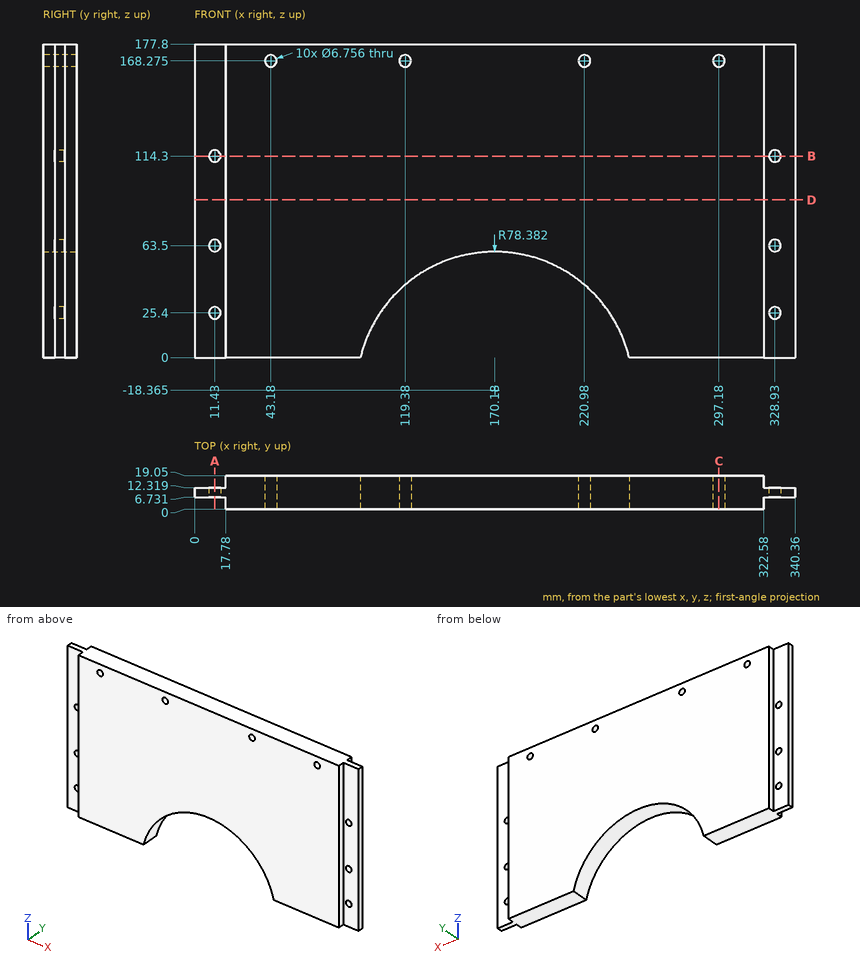
Here's the drawing with two shaded views (mm, measured from the low corner). I have some questions. Give positions to 0.01 mm unless a question says otherwise; leave off trailing zeros. Loops run counter-clockwise (first coordinate to the right, second up) from the corner with the lowest first, then second, coordinate; pieces in that order, holes last. Notation, with made-up numbers: (24.5, -10.5) -> (31.5, -10.5) arc R18 cw to (31.5, 4.5) -> close; hole circle Ø2 at (9, 16.25). An arc over 180 degrees is marked (long way). Answer as a JSON object with one key per item and string values. Group by question number.
Item 1: Imagine slicing it at A-A on x = 11.43. Write out the boundary of the cut face in (y, z).
Item 2: Imagine slicing it at C-C on x = 297.18. Write out the boundary of the cut face in (y, z).
Item 3: I need wall thicknesses on L1, parallel to Z at x = 328.93, y = 10.95; L2, parallel to Z at x = 297.18, y = 12; L3, parallel to X at y = 10, z = 167.5. Which ranges of each line are inside material? Lowest first, please.
Item 4: Imagine slicing it at B-B on z = 114.3. Write out the boundary of the cut face in (x, y).
Item 5: Will these pins go through, and if not, where does the flat tip stop? pin 1 (19.5 mm diameter, centred on x = 4.5, z = 94.5, fed in from +Y); pin 2 (3.5 mm diameter, centred on y = 15, z = 117.5, fed in from +X); pin 3 (2 mm diameter, centred on y = 3, z = 68, fed in from -X).
Item 6: Imagine slicing it at D-D on z = 89.5. Write out the boundary of the cut face in (x, y).
Answer list:
{
 "1": {"outline": "(6.73, 0) -> (12.32, 0) -> (12.32, 22.02) -> (6.73, 22.02) -> close; (6.73, 28.78) -> (12.32, 28.78) -> (12.32, 60.12) -> (6.73, 60.12) -> close; (6.73, 66.88) -> (12.32, 66.88) -> (12.32, 110.92) -> (6.73, 110.92) -> close; (6.73, 117.68) -> (12.32, 117.68) -> (12.32, 177.8) -> (6.73, 177.8) -> close"},
 "2": {"outline": "(0, 0) -> (19.05, 0) -> (19.05, 164.9) -> (0, 164.9) -> close; (0, 171.65) -> (19.05, 171.65) -> (19.05, 177.8) -> (0, 177.8) -> close"},
 "3": {"L1": "z = 0 to 22.02, 28.78 to 60.12, 66.88 to 110.92, 117.68 to 177.8", "L2": "z = 0 to 164.9, 171.65 to 177.8", "L3": "x = 0 to 39.89, 46.47 to 116.09, 122.67 to 217.69, 224.27 to 293.89, 300.47 to 340.36"},
 "4": {"outline": "(0, 6.73) -> (8.05, 6.73) -> (8.05, 12.32) -> (0, 12.32) -> close; (14.81, 6.73) -> (17.78, 6.73) -> (17.78, 0) -> (322.58, 0) -> (322.58, 6.73) -> (325.55, 6.73) -> (325.55, 12.32) -> (322.58, 12.32) -> (322.58, 19.05) -> (17.78, 19.05) -> (17.78, 12.32) -> (14.81, 12.32) -> close; (332.31, 6.73) -> (340.36, 6.73) -> (340.36, 12.32) -> (332.31, 12.32) -> close"},
 "5": {"pin 1": "stops at y = 12.32", "pin 2": "stops at x = 322.58", "pin 3": "stops at x = 17.78"},
 "6": {"outline": "(0, 6.73) -> (17.78, 6.73) -> (17.78, 0) -> (322.58, 0) -> (322.58, 6.73) -> (340.36, 6.73) -> (340.36, 12.32) -> (322.58, 12.32) -> (322.58, 19.05) -> (17.78, 19.05) -> (17.78, 12.32) -> (0, 12.32) -> close"}
}
